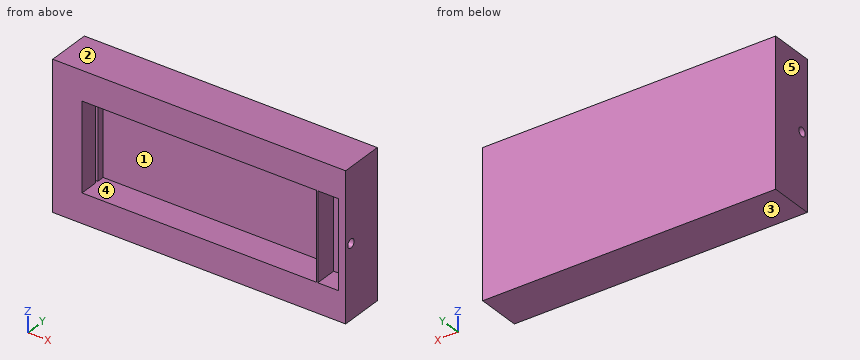
from build123d import *

# Parameters (mm, degrees)
SKETCH_1_W           = 20
SKETCH_1_H           = 10
EXTRUDE_1_DEPTH      = 3
SKETCH_2_W           = 16
SKETCH_2_H           = 6
CUT_EXTRUDE_1_DEPTH  = 2
SKETCH_3_W           = 6
SKETCH_3_H           = 0.2
CUT_EXTRUDE_2_DEPTH  = 1.5
SKETCH_5_W           = 1.3
SKETCH_5_H           = 6
CUT_EXTRUDE_4_DEPTH  = 1.3
SKETCH_11_R          = 0.3
CUT_EXTRUDE_7_DEPTH  = 0.5
SKETCH_14_W          = 1.4
SKETCH_14_H          = 6
CUT_EXTRUDE_9_DEPTH  = 1.5
CUT_EXTRUDE_START    = -0.5
SKETCH_15_R          = 0.3
CUT_EXTRUDE_10_DEPTH = 0.5


with BuildPart() as part:
    # 草图1 → 凸台-拉伸1 (new body)
    with BuildSketch(Plane(origin=(0, 0, 0), x_dir=(1, 0, 0), z_dir=(0, 1, 0))):
        Rectangle(SKETCH_1_W, SKETCH_1_H)
    extrude(amount=EXTRUDE_1_DEPTH)

    # 草图2 → 切除-拉伸1 (cut)
    with BuildSketch(Plane(origin=(0, 0, 0), x_dir=(1, 0, 0), z_dir=(0, 1, 0))):
        Rectangle(SKETCH_2_W, SKETCH_2_H)
    extrude(amount=CUT_EXTRUDE_1_DEPTH, mode=Mode.SUBTRACT)

    # 草图3 → 切除-拉伸2 (cut)
    with BuildSketch(Plane(origin=(-8, 0, 0), x_dir=(0, 0, -1), z_dir=(1, 0, 0))):
        with Locations((0, 1.4)):
            Rectangle(SKETCH_3_W, SKETCH_3_H)
    extrude(amount=-CUT_EXTRUDE_2_DEPTH, mode=Mode.SUBTRACT)

    # 草图5 → 切除-拉伸4 (cut)
    with BuildSketch(Plane.XZ.offset(-1.5)):
        with Locations((-8.85, 0)):
            Rectangle(SKETCH_5_W, SKETCH_5_H)
    extrude(amount=CUT_EXTRUDE_4_DEPTH, mode=Mode.SUBTRACT)

    # 草图11 → 切除-拉伸7 (cut)
    with BuildSketch(Plane.ZY.offset(10)):
        with Locations((0, 0.5)):
            Circle(SKETCH_11_R)
    extrude(amount=-CUT_EXTRUDE_7_DEPTH, mode=Mode.SUBTRACT)

    # 草图14 → 切除-拉伸9 (cut)
    with BuildSketch(Plane.XZ):
        with Locations((8.8, 0)):
            Rectangle(SKETCH_14_W, SKETCH_14_H)
    extrude(amount=-CUT_EXTRUDE_9_DEPTH, mode=Mode.SUBTRACT)

    # 草图15 → 切除-拉伸10 (cut)
    with BuildSketch(Plane(origin=(10, 0, 0), x_dir=(0, 0, -1), z_dir=(1, 0, 0)).offset(CUT_EXTRUDE_START)):
        with Locations(Location((0, 0.5, 0), (0, 0, 180))):
            Circle(SKETCH_15_R)
    extrude(amount=CUT_EXTRUDE_10_DEPTH, mode=Mode.SUBTRACT)


solid = part.part
The model under review builds one solid part; all positions refer to its coordinate system, in mm. Face numbers are marked on the shaded views. A direction names the side the tool comes from. Give positions to 0.01 mm unless a question says otherwise; leave off trailing zeros. Order: outer loops, then holes, each group sorted by start corner. A loop starts at its lowest first (then second) coordinate and runs counter-clockwise, first axis right, second up. Notation, with made-up numbers: M 42.25,-15 L 85.25,-15 A21 ccw 85.25,-5 Z; hole C 50,-38 d3. An arc over 180 degrees is marked long. One line per question, with ' | ' between items. Start each with the question number.
1) For the marked faces 1 and 2, list the 3-axis set-ups (+Z, -Z, +X, -X, +Y, -Y) from which the entire face can be reached by the end or side of a thin tool; tool diameter is ignored.
2) Clearance check with a flat-ended pin moving along its axis: P1, Ø3, axis at x = 3.5, z = 0, coming from the -Y side. State where the tip first meets the part, or that it passes through.
3) Mouldability with a two-part tool opening along X and no side actions: class the marked faces 3, 4 and 5 as pulls with the +X half, pulls with the -X half, needs draft (parallel to the pull), parting line crosses it, or undercut.
4) Consider section C-C, the plane z = 1. Give the boundary of the cut face in (x, y), then the cut area to 3 significant figures.
5) Consider section A-A, the plane y = 1.7. Give the boundary of the cut face in (x, z).
6) Wall thickness on L1, parallel to Y at x = -9, z = -2.75; L2, parallel to Z at x = -6.75, y = 0.5; L3, parallel to X at y = 1.9, z = 2.5: over which ranges is each line inside the solid? List them lowest first. Write a range as from..to.
7) Consider section B-B, the plane x = 3. Give the boundary of the cut face in (y, z), then the cut area to 3 significant figures.
Found:
1) face 1: -Y | face 2: +Z, +X, -X, +Y, -Y
2) P1: stops at y = 2
3) face 3: needs draft | face 4: undercut | face 5: pulls with the -X half
4) outline: M -10,0 L -8,0 L -8,1.3 L -8.2,1.3 L -8.2,0.2 L -9.5,0.2 L -9.5,1.5 L -8,1.5 L -8,2 L 8,2 L 8,0 L 8.1,0 L 8.1,1.5 L 9.5,1.5 L 9.5,0 L 10,0 L 10,3 L -10,3 Z | area: 24.2 mm²
5) outline: M -10,-5 L 10,-5 L 10,5 L -10,5 Z; hole M -8,-3 L 8,-3 L 8,3 L -8,3 Z
6) L1: y = 0..0.2, 1.5..3 | L2: z = -5..-3, 3..5 | L3: x = -10..-8, 8..10
7) outline: M 0,-5 L 3,-5 L 3,5 L 0,5 L 0,3 L 2,3 L 2,-3 L 0,-3 Z | area: 18.0 mm²
